Autodesk Inventor part; units mm, degrees
ref_plane "YZ Plane" through (0, 0, 0) normal (1, 0, 0) x (0, 1, 0)
ref_plane "XZ Plane" through (0, 0, 0) normal (0, 1, 0) x (-1, 0, 0)
ref_plane "XY Plane" through (0, 0, 0) normal (0, 0, 1) x (1, 0, 0)
sketch "Sketch1" plane through (0, 0, 0) normal (0, 0, 1) x (1, 0, 0)
  line L0 (-1.5, 0) -> (1.5, 0)
  line L1 (-2.5, -15) -> (2.5, -15)
  line L2 (-1.5, 0) -> (-2.5, -5)
  line L3 (1.5, 0) -> (2.5, -5)
  line L4 (1.5, -5) -> (1.5, -5)
  line L5 (-2.5, -10) -> (-1.5, -5)
  line L6 (1.5, -5) -> (2.5, -10)
  line L7 (-1.5, -10) -> (-1.5, -10)
  line L8 (1.5, -10) -> (2.5, -15)
  line L9 (-1.5, -10) -> (-2.5, -15)
  line L10 (1.5, -10) -> (2.5, -15)
  line L11 (0, 0) -> (0, -15)
  line L12 (-2.5, -10) -> (2.5, -10)
  line L13 (-2.5, -5) -> (2.5, -5)
  point P0 (0, -5)
  point P1 (0, -10)
  point P2 (0, -5)
  point P3 (0, -10)
  point P4 (1.9444, -10)
  dimension "d1" = 5
  dimension "d5" = 5
  dimension "d15" = 5
  dimension "d16" = 1.5
  dimension "d17" = 1.5
  dimension "d18" = 1.5
  dimension "d19" = 1.5
  dimension "d20" = 5
  dimension "d21" = 5
  dimension "d22" = 5
revolve "Revolution1" add sketch "Sketch1" angle 360 about axis through (0, 0, 0) along (0, -1, 0) contours L0 L3 L13 L11 | L13 L6 L12 L11 | L12 L8 L1 L11
properties part number "Valve_Plug_V2"
Input: part model. Units: mm. Frame: model coordinates. A direction names the side the tool comes from. Round coordinates to 2 decimals unless told otherwise and drop trailing zeros. Loops run counter-clockwise (first coordinate to the right, second up) from the corner with the lowest first, then second, coordinate; pieces in that order, holes last.
1) Pull-direction query (Y, two-part tool) for faces 1 (the flat face through (0, -15, 0)), 2 (the flat face through (2, -10, 0)), 3 (the flat face through (0, 0, 0)); classes: released by +Y, released by -Y, zero draft, split by the parting line, or undercut.
Ans:
face 1: released by -Y
face 2: undercut
face 3: released by +Y
2) Pin query (flat end, axial travel): pin 1 (1 mm diameter, centred on x = 2, y = -8, fed in from -Z); pin 2 (1 mm diameter, centred on x = -1, y = -4, fed in from +Z). Return the tip coordinate at first contact, or that it passes through.
Ans:
pin 1: stops at z = -1.49
pin 2: stops at z = 2.28
3) Section query D-D on x = 1.75. Count the separate pieces of the cut face and the enclosed holes in it, plus the area to 3 significant figures.
Ans:
separate pieces: 3
enclosed holes: 0
area: 25.8 mm2
4) Section query B-B on x = 0. Return the cut outline in (y, z), plus the area to 3 significant figures.
Ans:
outline: (-15, -2.5) - (-10, -1.5) - (-10, -2.5) - (-5, -1.5) - (-5, -2.5) - (0, -1.5) - (0, 1.5) - (-5, 2.5) - (-5, 1.5) - (-10, 2.5) - (-10, 1.5) - (-15, 2.5) - close
area: 60.0 mm2
5) Section query C-C on y = -7.5. Return the cut outline in (x, z).
Ans:
outline: circle Ø4 at (0, 0)
6) Section query A-A on z = 0. Return the cut outline in (x, y).
Ans:
outline: (-2.5, -15) - (2.5, -15) - (1.5, -10) - (2.5, -10) - (1.5, -5) - (2.5, -5) - (1.5, 0) - (-1.5, 0) - (-2.5, -5) - (-1.5, -5) - (-2.5, -10) - (-1.5, -10) - close
7) Set-up query: faces 4 (the conical face through (0.875, -11.979, -1.682)), 5 (the conical face through (0.875, -1.979, -1.682)). Return all of +Z, -Z, +X, -X, +Y, -Y with unobstructed straight access to the full face (end or side cutting, diameter ignored); none if empty.
Ans:
face 4: none
face 5: +Y
8) Material intervals for line 1 (Z direction, x = -0.15, y = -12.75); line 2 (X direction, y = -7, z = -0.6); line 3 (X direction, y = -9.25, z = -1.3), sorted ascending.
Ans:
line 1: z = -2.04 to 2.04
line 2: x = -1.8 to 1.8
line 3: x = -1.96 to 1.96
